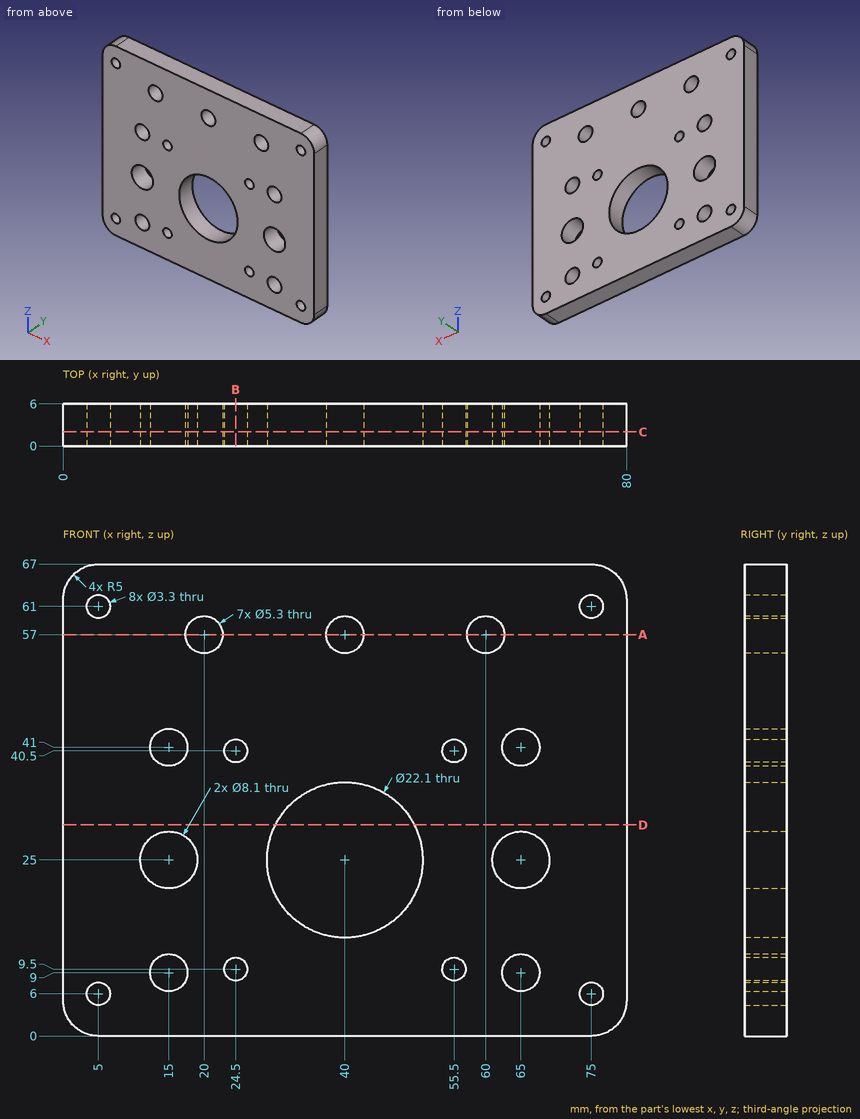
Input: dimensioned drawing with shaded views. Units: mm. Origin: part minimum x, y, z. Round coordinates to 2 decimals unless told otherwise and drop trailing zeros. Order: outer loops, then holes, each group sorted by start corner. A loop starts at its lowest first (then second) coordinate and runs counter-clockwise, first axis right, second up. Notation, with made-up numbers: (34, -16) - (56, -16) arc R12 cw to (56, -7) - close; hole circle Ø6 at (87, 78.25). An arc over 180 degrees is marked (long way). Use CSV: the item, a comma, the result in double quotes. Start each with the question number.
Q1. Material intervals for line 1 along X through (y, z) = (4.3, 57); line 2 along X through (y, z) = (2.7, 25); line 3 along Z through (x, y) = (65, 3.3), sorted ascending. Write a range as from..to.
Q2. Section query C-C (y = 2.05). State how many separate pieces and enclosed holes the cut face has, and give its area (3 significant figures).
Q3. Section query D-D (z = 30). Return loops of the section in (x, y), and give its area (3 significant figures).
Q4. Section query A-A (z = 57). Return loops of the section in (x, y), and give its area (3 significant figures).
Q5. Section query B-B (x = 24.5). Return loops of the section in (y, z), and give its area (3 significant figures).
Q6. First-contact query: pin 1 (3 mm diameter, centred on x = 65, z = 41, fed in from -Y). Flat tip, straight axial feed; report the tip coordinate or a pass-through.
Result set:
1,line 1,"x = 0..17.35, 22.65..37.35, 42.65..57.35, 62.65..80"
1,line 2,"x = 0..10.95, 19.05..28.95, 51.05..60.95, 69.05..80"
1,line 3,"z = 0..6.35, 11.65..20.95, 29.05..38.35, 43.65..67"
2,separate pieces,"1"
2,enclosed holes,"18"
2,area,"4,630 mm2"
3,outline,"(0, 0) - (30.15, 0) - (30.15, 6) - (0, 6) - close; (49.85, 0) - (80, 0) - (80, 6) - (49.85, 6) - close"
3,area,"362 mm2"
4,outline,"(0, 0) - (17.35, 0) - (17.35, 6) - (0, 6) - close; (22.65, 0) - (37.35, 0) - (37.35, 6) - (22.65, 6) - close; (42.65, 0) - (57.35, 0) - (57.35, 6) - (42.65, 6) - close; (62.65, 0) - (80, 0) - (80, 6) - (62.65, 6) - close"
4,area,"385 mm2"
5,outline,"(0, 0) - (6, 0) - (6, 7.85) - (0, 7.85) - close; (0, 11.15) - (6, 11.15) - (6, 38.85) - (0, 38.85) - close; (0, 42.15) - (6, 42.15) - (6, 67) - (0, 67) - close"
5,area,"362 mm2"
6,pin 1,"passes through"
